Geometry check sheet. Reference: the model listing, model coordinates, mm. Face numbers are marked on the shaded views. A direction names the side the tool comes from. Coordinates: 2 decimals unless noted, no trailing zeros. Loops run counter-clockwise (first coordinate to the right, second up) from the corner with the lowest first, then second, coordinate; pieces in that order, holes last. Notation, with made-up numbers: (83.25, 48.5) - (136.25, 48.5) arc R16 ccw to (136.25, 61.5) - close; hole circle Ø1 at (61.5, 75). An arc over 180 degrees is marked (long way). Write item = value, one per line. Start each with the question number.
Solid Edge part; units mm, degrees
sketch "Sketch1" plane through (0, 0, 0) normal (0, 0, 1) x (1, 0, 0)
  line L0 (25, 30) -> (-25, 30)
  line L1 (-25, 30) -> (-25, -30)
  line L2 (-25, -30) -> (25, -30)
  line L3 (25, -30) -> (25, 30)
extrude "Extrusionsausprägung_24" add sketch "Sketch1" against normal blind 5
sketch "Sketch2" plane through (0, 0, 0) normal (0, 0, 1) x (0, -1, 0)
  line L0 (-30, 15.5) -> (30, 15.5)
  line L1 (30, 15.5) -> (30, 25)
  line L2 (30, 25) -> (-30, 25)
  line L3 (-30, 25) -> (-30, 15.5)
extrude "Extrusionsausprägung_25" add sketch "Sketch2" along normal blind 4
mirror "Mirror1" about plane through (0, 0, 0) normal (1, 0, 0) of "Extrusionsausprägung_25"
sketch "Sketch3" plane through (0, 0, -5) normal (0, 0, -1) x (0, 1, 0)
  circle A0 centre (-23, 20) radius 3.3
  circle A1 centre (23, 20) radius 3.3
extrude "Extrusionsausschnitt_32" cut sketch "Sketch3" against normal blind 38
sketch "Sketch4" plane through (0, 0, -5) normal (0, 0, -1) x (0, 1, 0)
  circle A0 centre (0, 0) radius 9
extrude "Extrusionsausschnitt_33" cut sketch "Sketch4" against normal blind 1.6
mirror "Mirror2" about plane through (0, 0, 0) normal (1, 0, 0) of "Extrusionsausschnitt_32"
sketch "Sketch5" plane through (0, 0, -5) normal (0, 0, -1) x (0, 1, 0)
  circle A0 centre (0, 0) radius 10
  circle A1 centre (0, 0) radius 6.5
extrude "Extrusionsausprägung_27" add sketch "Sketch5" along normal blind 20
chamfer "Fase_14" distance 4 angle 45 1 edges at (0, -10, -5)
chamfer "Fase_15" distance 2 angle 45 1 edges at (0, -6.5, -25)
fillet "Verrundung_17" radius 2 8 edges at (-25, -30, -0.5) (-15.5, -30, 2) (15.5, -30, 2) (25, -30, -0.5) (-25, 30, -0.5) (25, 30, -0.5) (15.5, 30, 2) (-15.5, 30, 2)
chamfer "Fase_16" distance 0.5 angle 45 20 edges at (16.7, -23, 4) (16.7, 23, 4) (20.25, 30, 4) (16.0858, 29.4142, 4) (15.5, 0, 4) (16.0858, -29.4142, 4) (20.25, -30, 4) (24.4142, -29.4142, 4) (25, 0, 4) (24.4142, 29.4142, 4) (-16.7, 23, 4) (-16.7, -23, 4) (-15.5, 0, 4) (-16.0858, 29.4142, 4) (-20.25, 30, 4) (-24.4142, 29.4142, 4) (-25, 0, 4) (-24.4142, -29.4142, 4) (-20.25, -30, 4) (-16.0858, -29.4142, 4)
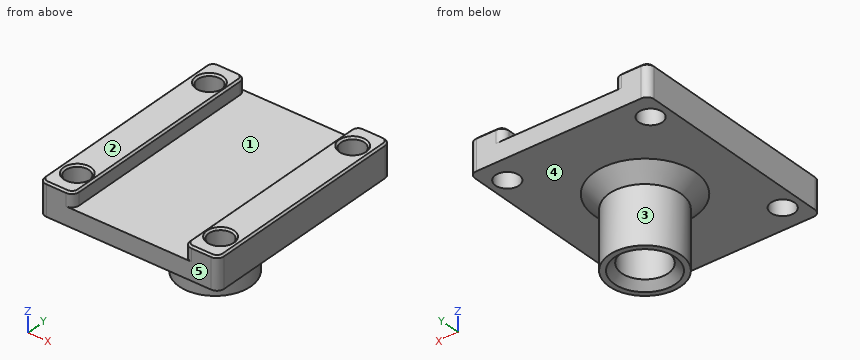
(1) Sectioned sample at B-B on y = -23. Enter the section's corners in (x, z), plus the area to 3 significant figures.
(2) Sectioned sample at A-A on z = -2.5. Enter the section's corners in (x, y), plus the area to 3 significant figures.
(3) Scan lines: line 1 (X direction, y = -23, z = 1.25); line 2 (X direction, y = -11, z = 0.25); line 3 (X direction, y = 0, z = -11). Record each from-to range of solid material in increasing order.
(4) Tool access check on the marked faces 4 and 5. Record the directions out of +Z, -Z, +X, -X, +Y, -Y that give a thin tool (end or side, any length) a straight path to the whole face; none if there is none.
(5) Draft check along X on the marked faces 1, 2 and 3. Enter one of: pulls with the +X half, pulls with the -X half, needs draft (parallel to the pull), parting line crosses it, or undercut.
(6) Sectioned sample at D-D on y = 0. Enter the section's corners in (x, z).
(7) Sectioned sample at C-C on x = 20. Enter the section's corners in (y, z).
(8) Depth check by flat-ended pin: pin 1 (12 mm diameter, centred on y = 12, z = -11.5, fed in from -X); pin 2 (17 mm diameter, centred on x = 0, y = 0, fed in from +Z); pin 3 (12 mm diameter, centred on x = -11.5, z = -20.5, fed in from -Y); pin 4 (4 mm diameter, centred on x = -20, y = -23, fed in from +Z). Enter the tip coordinate at first touch or a pass-through.
Working result:
q1.outline = (-25, -5) - (-23.3, -5) - (-23.3, 3.5) - (-23.8, 4) - (-24.5, 4) - (-25, 3.5) - close; (-16.7, -5) - (16.7, -5) - (16.7, 3.5) - (16.2, 4) - (16, 4) - (15.5, 3.5) - (15.5, 0) - (-15.5, 0) - (-15.5, 3.5) - (-16, 4) - (-16.2, 4) - (-16.7, 3.5) - close; (23.3, -5) - (25, -5) - (25, 3.5) - (24.5, 4) - (23.8, 4) - (23.3, 3.5) - close
q1.area = 206 mm2
q2.outline = (-25, -28) arc R2 ccw to (-23, -30) - (23, -30) arc R2 ccw to (25, -28) - (25, 28) arc R2 ccw to (23, 30) - (-23, 30) arc R2 ccw to (-25, 28) - close; hole circle Ø6.6 at (-20, -23); hole circle Ø6.6 at (-20, 23); hole circle Ø6.6 at (20, -23); hole circle Ø6.6 at (20, 23)
q2.area = 2,860 mm2
q3.line_1 = -25 to -23.3, -16.7 to -15.5, 15.5 to 16.7, 23.3 to 25
q3.line_2 = -25 to -15.5, 15.5 to 25
q3.line_3 = -10 to -6.5, 6.5 to 10
q4.face_4 = -Z
q4.face_5 = +Z, -Z, +X, -X, -Y
q5.face_1 = undercut
q5.face_2 = needs draft
q5.face_3 = parting line crosses it
q6.outline = (-25, -5) - (-14, -5) - (-10, -9) - (-10, -25) - (-8.5, -25) - (-6.5, -23) - (-6.5, -5) - (-9, -5) - (-9, -3.4) - (9, -3.4) - (9, -5) - (6.5, -5) - (6.5, -23) - (8.5, -25) - (10, -25) - (10, -9) - (14, -5) - (25, -5) - (25, 3.5) - (24.5, 4) - (16, 4) - (15.5, 3.5) - (15.5, 0) - (-15.5, 0) - (-15.5, 3.5) - (-16, 4) - (-24.5, 4) - (-25, 3.5) - close
q7.outline = (-30, -5) - (-26.3, -5) - (-26.3, 3.5) - (-26.8, 4) - (-29.5, 4) - (-30, 3.5) - close; (-19.7, -5) - (19.7, -5) - (19.7, 3.5) - (19.2, 4) - (-19.2, 4) - (-19.7, 3.5) - close; (26.3, -5) - (30, -5) - (30, 3.5) - (29.5, 4) - (26.8, 4) - (26.3, 3.5) - close
q8.pin_1 = -8.99
q8.pin_2 = 0
q8.pin_3 = -8.35
q8.pin_4 = through
